Verification items for the finished model (mm, model axes). A direction names the side the tool comes from. Coordinates: 2 decimals unless noted, no trailing zeros. Order: outer loops, then holes, each group sorted by start corner. A loop starts at its lowest first (then second) coordinate and runs counter-clockwise, first axis right, second up. Notation, with made-up numbers: (73, 7.5) - (100, 7.5) arc R13 ccw to (100, 31.5) - close; hole circle Ø2 at (72, 65.25). An arc over 180 degrees is marked (long way). Answer as CSV lines item,"result". Start each with the question number.
1. Material ranges on L1, parallel to X at y = 1.3, z = -19.05; L2, parallel to Y at x = 0, z = 12; L3, parallel to Y at x = 0, z = -9.5 (3 decimals), recorded low to high. Write a range as [from, to].
2. Section check C-C (x = 12). Record the cut outline in (y, z) (3 decimals), and give its area (3 significant figures).
3. Section check A-A (z = -19.05). Record the cut outline in (x, y) (3 decimals), and give its area (3 significant figures).
4. Go/stop test with flat-tipped pins: pin 1 (5.5 mm diameter, centred on x = 12.7, z = -19.05, fed in from +Y) (3 decimals); pin 2 (3.5 mm diameter, centred on y = 18.5, z = 10.5, fed in from -X) (3 decimals); pin 3 (1 mm diameter, centred on y = 20.5, z = 10.5, fed in from +X) (3 decimals). Record where each tip stops, or that it passes through.
5. Mould release check, pull along X, two halves, no side actions. Record for faces 5 (the cylindrical face through (12, 1.6, -17.5)), 6 (the cylindrical face through (11.7, 4.13, 11.09)), 7 (the flat face through (-10.795, 17, 11)): pulls with the +X half, pulls with the -X half, needs draft (parallel to the pull), parting line crosses it, or undercut.
6. Set-up check for faces 1 (the flat face through (0, 18, 9.525)), 2 (the flat face through (18, 21, 12.7)), 3 (the cylindrical face through (-11.75, 4.08, 11.09)), 4 (the cylindrical face through (-0.237, 39.367, 11.135)): record each of +Z, -Z, +X, -X, +Y, -Y from which the full face is reachable in a straight line by a thin tool's end or side.
7. Section check D-D (y = 14). Record the cut outline in (x, z) (3 decimals).
from build123d import *

# Parameters (mm, degrees)
BOSS_EXTRUDE1_DEPTH  = 3.175
M3_CLEARANCE_HOLE1_D = 3.4
SKETCH7_W            = 50.8
SKETCH7_H            = 3.175
BOSS_EXTRUDE3_DEPTH  = 39.37
BOSS_EXTRUDE4_DEPTH  = 3.175
SKETCH9_R            = 8.73125
CUT_EXTRUDE1_DEPTH   = 7.35
FILLET1_R            = 3.175


with BuildPart() as part:
    # Sketch2 → Boss-Extrude1 (new body)
    with BuildSketch(Plane(origin=(0, 0, 0), x_dir=(1, 0, 0), z_dir=(0, 1, 0))):
        Polygon((-25.4, -12.7), (25.4, -12.7), (25.4, 12.7), (25.4, 25.4), (-25.4, 25.4), (-25.4, 12.7), align=None)
    extrude(amount=BOSS_EXTRUDE1_DEPTH)

    # M3 Clearance Hole1 (through all)
    with Locations(Plane(origin=(-12.7, 0, -19.05), x_dir=(0, 0, -1), z_dir=(0, -1, 0))):
        with Locations((0, 0), (0, 25.4)):
            Hole(M3_CLEARANCE_HOLE1_D / 2)

    # Sketch7 → Boss-Extrude3 (add)
    with BuildSketch(Plane.XZ):
        with Locations((0, 14.2875)):
            Rectangle(SKETCH7_W, SKETCH7_H)
    extrude(amount=-BOSS_EXTRUDE3_DEPTH)

    # Sketch8 → Boss-Extrude4 (add)
    with BuildSketch(Plane(origin=(0, 0, 12.7), x_dir=(-1, 0, 0), z_dir=(0, 0, -1))):
        with BuildLine():
            Line((-10.795, 28.575), (-10.795, 3.175))
            Line((-10.795, 3.175), (10.795, 3.175))
            Line((10.795, 3.175), (10.795, 28.575))
            ThreePointArc((10.795, 28.575), (0, 39.37), (-10.795, 28.575))
        make_face()
    extrude(amount=BOSS_EXTRUDE4_DEPTH)

    # Sketch9 → Cut-Extrude1 (cut, through all)
    with BuildSketch(Plane(origin=(0, 0, 9.525), x_dir=(-1, 0, 0), z_dir=(0, 0, -1))):
        with Locations((0, 28.575)):
            Circle(SKETCH9_R)
    extrude(amount=-CUT_EXTRUDE1_DEPTH, mode=Mode.SUBTRACT)

    # Fillet1
    fillet1_edges = [part.edges().sort_by_distance(p)[0] for p in [
        (10.795, 3.175, 11.1125),
        (-10.795, 3.175, 11.1125),
    ]]
    fillet(fillet1_edges, radius=FILLET1_R)


solid = part.part
Evaluation:
1,L1,"x = [-25.4, -14.4], [-11, 11], [14.4, 25.4]"
1,L2,"y = [0, 19.84], [37.31, 39.37]"
1,L3,"y = [0, 3.175]"
2,outline,"(0, -25.4) - (3.175, -25.4) - (3.175, -20.599) - (0, -20.599) - close; (0, -17.501) - (3.175, -17.501) - (3.175, 9.525) - (3.86, 9.525) - (3.86, 12.7) - (39.37, 12.7) - (39.37, 15.875) - (0, 15.875) - close"
2,area,"238 mm²"
3,outline,"(-25.4, 0) - (-14.4, 0) - (-14.4, 3.175) - (-25.4, 3.175) - close; (-11, 0) - (11, 0) - (11, 3.175) - (-11, 3.175) - close; (14.4, 0) - (25.4, 0) - (25.4, 3.175) - (14.4, 3.175) - close"
3,area,"140 mm²"
4,pin 1,"stops at y = 3.175"
4,pin 2,"stops at x = -10.795"
4,pin 3,"stops at x = 10.795"
5,face 5,"undercut"
5,face 6,"pulls with the +X half"
5,face 7,"pulls with the -X half"
6,face 1,"-Z, +X, -X, +Y"
6,face 2,"-Z, +X, +Y"
6,face 3,"-Z, -X, +Y"
6,face 4,"-Z, +Y"
7,outline,"(-25.4, 12.7) - (-10.795, 12.7) - (-10.795, 9.525) - (10.795, 9.525) - (10.795, 12.7) - (25.4, 12.7) - (25.4, 15.875) - (-25.4, 15.875) - close"
